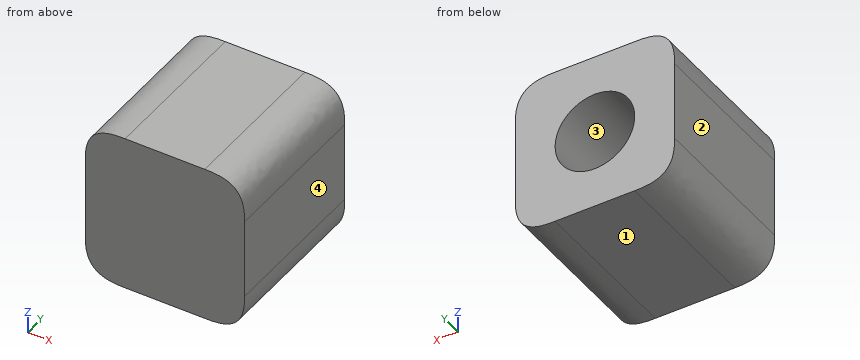
```python
from build123d import *

# Parameters (mm, degrees)
SKETCH2_W           = 8
SKETCH2_H           = 8
SKETCH2_R           = 2
BOSS_EXTRUDE1_DEPTH = 7
SKETCH3_W           = 8
SKETCH3_H           = 8
BOSS_EXTRUDE2_DEPTH = 1
FILLET1_SIZE        = 2


with BuildPart() as part:
    # Sketch2 → Boss-Extrude1 (new body)
    with BuildSketch(Plane(origin=(0, 0, 0), x_dir=(1, 0, 0), z_dir=(0, 1, 0))):
        Rectangle(SKETCH2_W, SKETCH2_H)
        with Locations(Location((0, 0, 0), (0, 0, 270))):
            Circle(SKETCH2_R, mode=Mode.SUBTRACT)
    extrude(amount=BOSS_EXTRUDE1_DEPTH)

    # Sketch3 → Boss-Extrude2 (add)
    with BuildSketch(Plane.XZ):
        Rectangle(SKETCH3_W, SKETCH3_H)
    extrude(amount=BOSS_EXTRUDE2_DEPTH)

    # Fillet1
    # a fillet whose section is not a circle: 2 mm, written as the material it takes off along each edge
    with BuildSketch(Plane(origin=(4, -6, 4), x_dir=(-1, 0, 0), z_dir=(0, 1, 0)), Plane(origin=(-4, 12, 4), x_dir=(1, 0, 0), z_dir=(0, -1, 0))) as fillet1_piece_1:
        with BuildLine():
            add(Edge.make_bspline([(FILLET1_SIZE, 0), (FILLET1_SIZE * 0.831801948466, 0), (FILLET1_SIZE * 0.663603896932, 0), (FILLET1_SIZE * 0.292893218813, -FILLET1_SIZE * 0.0716919198361), (FILLET1_SIZE * 0.0716919198361, -FILLET1_SIZE * 0.292893218813), (0, -FILLET1_SIZE * 0.663603896932), (0, -FILLET1_SIZE * 0.831801948466), (0, -FILLET1_SIZE)], knots=[0, 0, 0, 0, 0, 0, 0.5, 0.5, 1, 1, 1, 1, 1, 1], degree=5))
            Line((0, -FILLET1_SIZE), (0, 0))
            Line((0, 0), (FILLET1_SIZE, 0))
        make_face()
    extrude(amount=18, mode=Mode.SUBTRACT)
    with BuildSketch(Plane(origin=(-4, 12, -4), x_dir=(1, 0, 0), z_dir=(0, -1, 0)), Plane(origin=(4, -6, -4), x_dir=(-1, 0, 0), z_dir=(0, 1, 0))) as fillet1_piece_2:
        with BuildLine():
            add(Edge.make_bspline([(FILLET1_SIZE, 0), (FILLET1_SIZE * 0.831801948466, 0), (FILLET1_SIZE * 0.663603896932, 0), (FILLET1_SIZE * 0.292893218813, FILLET1_SIZE * 0.0716919198361), (FILLET1_SIZE * 0.0716919198361, FILLET1_SIZE * 0.292893218813), (0, FILLET1_SIZE * 0.663603896932), (0, FILLET1_SIZE * 0.831801948466), (0, FILLET1_SIZE)], knots=[0, 0, 0, 0, 0, 0, 0.5, 0.5, 1, 1, 1, 1, 1, 1], degree=5))
            Line((0, FILLET1_SIZE), (0, 0))
            Line((0, 0), (FILLET1_SIZE, 0))
        make_face()
    extrude(amount=18, mode=Mode.SUBTRACT)


solid = part.part
```
Source: CAD feature listing. Evaluate the final solid. Frame: model axes, mm. Face numbers are marked on the shaded views. Round coordinates to 2 decimals unless told otherwise and drop trailing zeros. Write each loop counter-clockwise with the first axis right and the second up, starting at its lowest first coordinate (ties: lowest second). Pieces come first, ordered by that corner, then holes. Notation, with made-up numbers: M 54,71 L 88,71 A29 ccw 88,107 Z; hole C -6,5 d11. An arc over 180 degrees is marked long. Use CSV: the item, a comma, the result in double quotes. Start each with the question number.
Q1. Cut plane A-A on x = 0. Output: boundary loops of the cut face in (y, z).
Q2. Line query: line 1 (X direction, y = 2.5, z = 0); line 2 (X direction, y = 1, z = -1); line 3 (Z direction, x = 0.25, y = 0.75). Output: solid intervals per line, ascending. Write a range as from..to.
Q3. Cut plane B-B on z = 0. Output: boundary loops of the cut face in (x, y), plus the area to 3 significant figures.
Q4. Pull-direction query (X, two-part tool) for the marked faces 1, 2, 3 and 4; classes: +X half, -X half, draft (parallel to the pull), parting line (faces both ways), or undercut.
Q5. First-contact query: P1, Ø2.5, axis at x = 0, z = 0, coming from the +Y side. Flat tip, straight axial feed; report the tip coordinate or a pass-through.
Results found:
1,outline,"M -1,-4 L 7,-4 L 7,-2 L 0,-2 L 0,2 L 7,2 L 7,4 L -1,4 Z"
2,line 1,"-4..-2, 2..4"
2,line 2,"-4..-1.73, 1.73..4"
2,line 3,"-4..-1.98, 1.98..4"
3,outline,"M -4,-1 L 4,-1 L 4,7 L 2,7 L 2,0 L -2,0 L -2,7 L -4,7 Z"
3,area,"36.0 mm^2"
4,face 1,"draft"
4,face 2,"-X half"
4,face 3,"undercut"
4,face 4,"+X half"
5,P1,"y = 0"
